from build123d import *

# Parameters (mm, degrees)
EXTRUDE_1_DEPTH   = 11
SKETCH_1_R        = 5
EXTRUDE_1_2_DEPTH = 11
EXTRUDE_1_3_DEPTH = 11
SKETCH_2_W        = 30
SKETCH_2_H        = 10
EXTRUDE_2_DEPTH   = 4
SKETCH_3_R        = 5
EXTRUDE_3_DEPTH   = 11
SKETCH_4_W        = 30
SKETCH_4_H        = 10
EXTRUDE_4_DEPTH   = 4
SKETCH_5_W        = 30
SKETCH_5_H        = 4
EXTRUDE_5_DEPTH   = 5
SKETCH_6_W        = 1.3
SKETCH_6_H        = 0.65
EXTRUDE_6_DEPTH   = 4


with BuildPart() as part:
    # Sketch 1 → Extrude 1 (new body)
    with BuildSketch(Plane(origin=(0, 0, 0), x_dir=(1, 0, 0), z_dir=(0, 1, 0))):
        with BuildLine():
            Line((0, 10), (0, 0))
            Line((0, 0), (5.202041029, 0))
            ThreePointArc((5.202041029, 0), (4, 5), (5.202041029, 10))
            Line((5.202041029, 10), (0, 10))
        make_face()
    extrude(amount=EXTRUDE_1_DEPTH)



with BuildPart() as body_2:
    # Sketch 1 → Extrude 1 2 (new body)
    with BuildSketch(Plane(origin=(0, 0, 0), x_dir=(1, 0, 0), z_dir=(0, 1, 0))):
        with Locations(Location((15, 5, 0), (0, 0, 270))):
            Circle(SKETCH_1_R)
    extrude(amount=EXTRUDE_1_2_DEPTH)


with BuildPart() as body_3:
    # Sketch 1 → Extrude 1 3 (new body)
    with BuildSketch(Plane(origin=(0, 0, 0), x_dir=(1, 0, 0), z_dir=(0, 1, 0))):
        with BuildLine():
            ThreePointArc((26, 5), (25.695268783, 2.428769622), (24.797958971, 0))
            Line((24.797958971, 0), (30, 0))
            Line((30, 0), (30, 10))
            Line((30, 10), (24.797958971, 10))
            ThreePointArc((24.797958971, 10), (25.695268783, 7.571230378), (26, 5))
        make_face()
    extrude(amount=EXTRUDE_1_3_DEPTH)


with BuildPart() as part_1:
    add(part.part)

    add(body_2.part)  # Extrude 2 merges body 2

    add(body_3.part)  # Extrude 2 merges body 3
    # Sketch 2 → Extrude 2 (add)
    with BuildSketch(Plane.XZ):
        with Locations((15, -5)):
            Rectangle(SKETCH_2_W, SKETCH_2_H)
    extrude(amount=EXTRUDE_2_DEPTH)

    # Sketch 3 → Extrude 3 (add)
    with BuildSketch(Plane(origin=(0, 11, 0), x_dir=(1, 0, 0), z_dir=(0, 1, 0))):
        with Locations(Location((15, 5, 0), (0, 0, 270))):
            Circle(SKETCH_3_R)
        with BuildLine():
            Line((24.797958971, 0), (30, 0))
            Line((30, 0), (30, 10))
            Line((30, 10), (24.797958971, 10))
            ThreePointArc((24.797958971, 10), (26, 5), (24.797958971, 0))
        make_face()
        with BuildLine():
            Line((5.202041029, 10), (0, 10))
            Line((0, 10), (0, 0))
            Line((0, 0), (5.202041029, 0))
            ThreePointArc((5.202041029, 0), (4, 5), (5.202041029, 10))
        make_face()
    extrude(amount=EXTRUDE_3_DEPTH)

    # Sketch 4 → Extrude 4 (add)
    with BuildSketch(Plane(origin=(0, 22, 0), x_dir=(1, 0, 0), z_dir=(0, 1, 0))):
        with Locations((15, 5)):
            Rectangle(SKETCH_4_W, SKETCH_4_H)
    extrude(amount=EXTRUDE_4_DEPTH)

    # Sketch 5 → Extrude 5 (add)
    with BuildSketch(Plane.XY):
        with Locations((15, 24)):
            Rectangle(SKETCH_5_W, SKETCH_5_H)
        with Locations((15, -2)):
            Rectangle(SKETCH_5_W, SKETCH_5_H)
    extrude(amount=EXTRUDE_5_DEPTH)

    # Sketch 6 → Extrude 6 (add)
    with BuildSketch(Plane.XY.offset(5)):
        with Locations((6.4, 24)):
            Rectangle(SKETCH_6_W, SKETCH_6_H)
        with Locations((2.1, 24)):
            Rectangle(SKETCH_6_W, SKETCH_6_H)
        with Locations((10.7, 24)):
            Rectangle(SKETCH_6_W, SKETCH_6_H)
        with Locations((15, 24)):
            Rectangle(SKETCH_6_W, SKETCH_6_H)
        with Locations((19.3, 24)):
            Rectangle(SKETCH_6_W, SKETCH_6_H)
        with Locations((23.6, 24)):
            Rectangle(SKETCH_6_W, SKETCH_6_H)
        with Locations((27.9, 24)):
            Rectangle(SKETCH_6_W, SKETCH_6_H)
        with Locations((6.4, -2)):
            Rectangle(SKETCH_6_W, SKETCH_6_H)
        with Locations((2.1, -2)):
            Rectangle(SKETCH_6_W, SKETCH_6_H)
        with Locations((10.7, -2)):
            Rectangle(SKETCH_6_W, SKETCH_6_H)
        with Locations((23.6, -2)):
            Rectangle(SKETCH_6_W, SKETCH_6_H)
        with Locations((19.3, -2)):
            Rectangle(SKETCH_6_W, SKETCH_6_H)
        with Locations((27.9, -2)):
            Rectangle(SKETCH_6_W, SKETCH_6_H)
    extrude(amount=EXTRUDE_6_DEPTH)


solid = part_1.part
Build history of the part. All positions in model axes, mm. A direction names the side the tool comes from. Round coordinates to 2 decimals unless told otherwise and drop trailing zeros. Write each loop counter-clockwise with the first axis right and the second up, starting at its lowest first coordinate (ties: lowest second). Pieces come first, ordered by that corner, then holes. Notation, with made-up numbers: M 44.5,57 L 100.5,57 A17 ccw 100.5,88 Z; hole C 74,37.5 d4. An arc over 180 degrees is marked long. Answer as a JSON object with one key per item and string values. Group by question number.
(1) Mould opens along Y. For faces 4 (the flat face through (28, -2.325, 7)), 5 (the flat face through (11, -1.675, 7)), 6 (the flat face through (11, 24.325, 7)) say: pulls with the +Y half, pulls with the -Y half, needs draft (parallel to the pull), parting line crosses it, or undercut.
(2) Cut at A-A (z = 1.5). Give the cut face in (x, y).
(3) Cut at B-B (y = 15.5). Give the cut face in (x, z), and give its area (3 significant figures).
(4) Which spindle directions (+Z, -Z, +X, -X, +Y, -Y) get a long thin tool onto all of the face, cutting with end or side? Do faces 1 (the flat face through (2, 24.325, 7)), 2 (the flat face through (19, -2.325, 7)), 3 (the flat face through (2, 23.675, 7)). Say none if no direction does.
(5) Drill centre lines: L1, parallel to X at y = 9.75, z = -5.25; L2, parallel to Y at x = 6.75, z = -5.25; L3, parallel to Y at x = 28.5, z = 5.75 (3 decimals). Where is each one in solid material? Low to high.
(6) Cut at C-C (x = 27.75). Give the cut face in (y, z) (3 decimals).
(7) Flat gauge pins, fed straight in: pin 1 (0.7 mm diameter, centred on y = -2, z = 8, fed in from +X); pin 2 (1 mm diameter, centred on x = 28, z = 6, fed in from -Y) (3 decimals); pin 3 (1.4 mm diameter, centred on x = 19, z = 7, fed in from +Y) (3 decimals). Where does each tip first touch, or does it go through?
(8) Cut at D-D (z = -4). Give the cut face in (x, y), and give its area (3 significant figures).
Responses:
{
 "1": {"face 4": "pulls with the -Y half", "face 5": "undercut", "face 6": "pulls with the +Y half"},
 "2": {"outline": "M 0,-4 L 30,-4 L 30,0 L 0,0 Z; M 0,22 L 30,22 L 30,26 L 0,26 Z"},
 "3": {"outline": "M 0,-10 L 5.2,-10 A11 cw 5.2,0 L 0,0 Z; C 15,-5 d10; M 24.8,-10 L 30,-10 L 30,0 L 24.8,0 A11 cw Z", "area": "166 mm2"},
 "4": {"face 1": "+Z, +X, -X, +Y", "face 2": "+Z, +X, -X, -Y", "face 3": "+Z, +X, -X"},
 "5": {"L1": "x = 0 to 4, 10.01 to 19.99, 26 to 30", "L2": "y = -4 to 0, 22 to 26", "L3": "y = -2.325 to -1.675, 23.675 to 24.325"},
 "6": {"outline": "M -4,-10 L 26,-10 L 26,5 L 24.325,5 L 24.325,9 L 23.675,9 L 23.675,5 L 22,5 L 22,0 L 0,0 L 0,5 L -1.675,5 L -1.675,9 L -2.325,9 L -2.325,5 L -4,5 Z"},
 "7": {"pin 1": "stops at x = 28.55", "pin 2": "stops at y = -2.325", "pin 3": "stops at y = 24.325"},
 "8": {"outline": "M 0,-4 L 30,-4 L 30,26 L 0,26 Z; hole M 4.05,0 L 10.1,0 L 10.1,22 L 4.05,22 Z; hole M 19.9,0 L 25.95,0 L 25.95,22 L 19.9,22 Z", "area": "634 mm2"}
}
